```python
from build123d import *

# Parameters (mm, degrees)
SKETCH3_W           = 28.2
SKETCH3_H           = 29.2
BOSS_EXTRUDE1_DEPTH = 3
BOSS_EXTRUDE2_START = 3
SKETCH3_3_W         = 28.2
SKETCH3_3_H         = 29.2
BOSS_EXTRUDE2_DEPTH = 30
SKETCH6_4_W         = 10.2
SKETCH6_4_H         = 20.4
CUT_EXTRUDE2_DEPTH  = 30
SKETCH8_R           = 2
CUT_EXTRUDE3_DEPTH  = 30


with BuildPart() as part:
    # Sketch3 → Boss-Extrude1 (new body)
    with BuildSketch(Plane(origin=(0, 0, 0), x_dir=(0, 0, -1), z_dir=(1, 0, 0))):
        with Locations((-1, 0)):
            Rectangle(SKETCH3_W, SKETCH3_H)
    extrude(amount=BOSS_EXTRUDE1_DEPTH)

    # Sketch3<3> → Boss-Extrude2 (add)
    with BuildSketch(Plane(origin=(0, 0, 0), x_dir=(0, 0, -1), z_dir=(1, 0, 0)).offset(BOSS_EXTRUDE2_START)):
        with Locations((-1, 0)):
            Rectangle(SKETCH3_3_W, SKETCH3_3_H)
        with BuildLine():
            Line((-10.1, 2.9), (-10.1, 9))
            ThreePointArc((-10.1, 9), (-9.777817459, 9.777817459), (-9, 10.1))
            Line((-9, 10.1), (-2.9, 10.1))
            Line((-2.9, 10.1), (-2.9, 7.9))
            Line((-2.9, 7.9), (-4.9, 7.9))
            Line((-4.9, 7.9), (-4.9, 5.749))
            Line((-4.9, 5.749), (-2.7515, 3.6005))
            Line((-2.7515, 3.6005), (2.7515, 3.6005))
            Line((2.7515, 3.6005), (4.9, 5.749))
            Line((4.9, 5.749), (4.9, 7.9))
            Line((4.9, 7.9), (2.9, 7.9))
            Line((2.9, 7.9), (2.9, 10.1))
            Line((2.9, 10.1), (9, 10.1))
            ThreePointArc((9, 10.1), (9.777817459, 9.777817459), (10.1, 9))
            Line((10.1, 9), (10.1, 2.9))
            Line((10.1, 2.9), (7.9, 2.9))
            Line((7.9, 2.9), (7.9, 4.9))
            Line((7.9, 4.9), (5.749, 4.9))
            Line((5.749, 4.9), (3.6005, 2.7515))
            Line((3.6005, 2.7515), (3.6005, -2.7515))
            Line((3.6005, -2.7515), (5.749, -4.9))
            Line((5.749, -4.9), (7.9, -4.9))
            Line((7.9, -4.9), (7.9, -2.9))
            Line((7.9, -2.9), (10.1, -2.9))
            Line((10.1, -2.9), (10.1, -9))
            ThreePointArc((10.1, -9), (9.777817459, -9.777817459), (9, -10.1))
            Line((9, -10.1), (2.9, -10.1))
            Line((2.9, -10.1), (2.9, -7.9))
            Line((2.9, -7.9), (4.9, -7.9))
            Line((4.9, -7.9), (4.9, -5.749))
            Line((4.9, -5.749), (2.7515, -3.6005))
            Line((2.7515, -3.6005), (-2.7515, -3.6005))
            Line((-2.7515, -3.6005), (-4.9, -5.749))
            Line((-4.9, -5.749), (-4.9, -7.9))
            Line((-4.9, -7.9), (-2.9, -7.9))
            Line((-2.9, -7.9), (-2.9, -10.1))
            Line((-2.9, -10.1), (-9, -10.1))
            ThreePointArc((-9, -10.1), (-9.777817459, -9.777817459), (-10.1, -9))
            Line((-10.1, -9), (-10.1, -2.9))
            Line((-10.1, -2.9), (-7.9, -2.9))
            Line((-7.9, -2.9), (-7.9, -4.9))
            Line((-7.9, -4.9), (-5.749, -4.9))
            Line((-5.749, -4.9), (-3.6005, -2.7515))
            Line((-3.6005, -2.7515), (-3.6005, 2.7515))
            Line((-3.6005, 2.7515), (-5.749, 4.9))
            Line((-5.749, 4.9), (-7.9, 4.9))
            Line((-7.9, 4.9), (-7.9, 2.9))
            Line((-7.9, 2.9), (-10.1, 2.9))
        make_face(mode=Mode.SUBTRACT)
    extrude(amount=BOSS_EXTRUDE2_DEPTH)

    # Sketch6 → section 1 of loft2
    with BuildSketch(Plane(origin=(0, 0, -43.1), x_dir=(-1, 0, 0), z_dir=(0, 0, -1)), mode=Mode.PRIVATE) as loft2_s1:
        with BuildLine():
            Line((-29.5, -14.6), (-3.5, -14.6))
            Line((-3.5, -14.6), (-3.5, 11.4))
            Line((-3.5, 11.4), (-29.5, 11.4))
            Line((-29.5, 11.4), (-29.5, -14.6))
        make_face()
    # loft from a face of the part (loft2)
    loft([part.faces().sort_by_distance((16.5, 0, -13.1))[0], loft2_s1.sketch])

    # Sketch6<4> → Cut-Extrude2 (cut)
    with BuildSketch(Plane(origin=(0, 0, -43.1), x_dir=(-1, 0, 0), z_dir=(0, 0, -1))):
        with Locations((-21.6, -1.6)):
            Rectangle(SKETCH6_4_W, SKETCH6_4_H)
        with Locations((-11.4, -1.6)):
            Rectangle(SKETCH6_4_W, SKETCH6_4_H)
    extrude(amount=-CUT_EXTRUDE2_DEPTH, mode=Mode.SUBTRACT)

    # Sketch8 → Cut-Extrude3 (cut)
    with BuildSketch(Plane(origin=(0, -11.8, 0), x_dir=(1, 0, 0), z_dir=(0, 1, 0))):
        with Locations(Location((16.5, 35.6, 0), (0, 0, 270))):
            Circle(SKETCH8_R)
        with Locations(Location((16.5, 20.6, 0), (0, 0, 270))):
            Circle(SKETCH8_R)
    extrude(amount=-CUT_EXTRUDE3_DEPTH, mode=Mode.SUBTRACT)

    # Mirror2: part across plane


with BuildPart() as part_1:
    add(part.part)
    add(part.part.mirror(Plane(origin=(3, 0, 15.1), x_dir=(1, 0, 0), z_dir=(0, 0, -1))))


solid = part_1.part
```
Build history of the part. All positions in model axes, mm. Coordinates: 2 decimals unless noted, no trailing zeros. Order: outer loops, then holes, each group sorted by start corner. A loop starts at its lowest first (then second) coordinate and runs counter-clockwise, first axis right, second up. Notation, with made-up numbers: (-21, -33.5) -> (-11, -33.5) arc R13 cw to (-11, -22.5) -> close; hole circle Ø11 at (-23.5, -31.75). An arc over 180 degrees is marked (long way). Answer in a Markdown table with one row per item. Add a question column.
Q1. Band-saw the part on B-B, the plane x = 5. Give the number of separate pieces and of enclosed holes in the cut face, then the cut area to 3 significant figures.
Q2. Band-saw the part on A-A, the plane z = 31. List the corners of the cut face in (x, y).
Q3. Drop flat-ended pins along their axis: pin 1 (2.5 mm diameter, centred on x = 24, y = -7, fed in from +Z); pin 2 (1 mm diameter, centred on x = 11, y = 4, fed in from -Z). Give the stop position or say it passes through.
Q4. Mould opens along Y. For faces 1 (the face through (27, -1, 73.3)), 2 (the face through (18, -10.1, 36)) say: +Y half, -Y half, draft (parallel to the pull), parting line (faces both ways), or undercut.
Q5. Wall check: line 1 along Z through (x, y) = (27, 2.75); line 2 along Z through (x, y) = (8, 9); line 3 along Y through (x, z) = (24, 21). Give the ranges that are in metal, low to high. Write a range as [from, to].
Answers follow:
| question | item | result |
|---|---|---|
| 1 | separate pieces | 1 |
| 1 | enclosed holes | 2 |
| 1 | area | 2,890 mm^2 |
| 2 | outline | (0, -14.6) -> (33, -14.6) -> (33, -3.6) -> (3, -3.6) -> (3, 3.6) -> (33, 3.6) -> (33, 14.6) -> (0, 14.6) -> close |
| 3 | pin 1 | z = 43.3 |
| 3 | pin 2 | z = -13.1 |
| 4 | face 1 | draft |
| 4 | face 2 | undercut |
| 5 | line 1 | [-43.1, -3.6], [3.6, 26.6], [33.8, 73.3] |
| 5 | line 2 | [-43.1, -10.1], [-2.9, 2.9], [10.1, 20.1], [27.3, 33.1], [40.3, 73.3] |
| 5 | line 3 | [-14.6, -10.08], [-2.9, 2.9], [10.08, 14.6] |
